For this review, take the finished solid that the model builds, in its own axes (mm). Face numbers are marked on the shaded views. Round coordinates to 2 decimals unless told otherwise and drop trailing zeros. Loops run counter-clockwise (first coordinate to the right, second up) from the corner with the lowest first, then second, coordinate; pieces in that order, holes last.
```python
from build123d import *

# Parameters (mm, degrees)
F0_R      = 0.381
F1_DEPTH  = 6.096
F2_SIZE2  = 0.3666174209
F2_SIZE   = 0.635
F0_R_2    = 1.1811
F1_FACE_R = 0.381
F3_DEPTH  = 0.762
F4_R      = 0.762
F4_R_2    = 0.508
F5_DEPTH  = 2.413
F6_R      = 1.1811
F6_R_2    = 0.762
F6_R_3    = 0.508
F7_DEPTH  = 0.762


with BuildPart() as f1:
    # F0 (on Top) → F1 (new body)
    with BuildSketch(Plane.XY):
        Circle(F0_R)
    extrude(amount=-F1_DEPTH)

    # F2
    f2_edges = [f1.edges().sort_by_distance(p)[0] for p in [
        (-0.381, 0, -6.096),
    ]]
    f2_side = f1.faces().sort_by_distance((-0.381, 0, -3.048))[0]
    chamfer(f2_edges, length=F2_SIZE, length2=F2_SIZE2, reference=f2_side)

    # F0 (on Top) + F1_face (on face) → F3 (join)
    with BuildSketch(Plane.XY):
        Circle(F0_R_2)
        Circle(F0_R, mode=Mode.SUBTRACT)
    with BuildSketch(Plane.XY):
        Circle(F1_FACE_R)
    extrude(amount=F3_DEPTH)

    # F4 (on face) → F5 (join)
    with BuildSketch(Plane.XY.offset(0.762)):
        Circle(F4_R)
        Circle(F4_R_2, mode=Mode.SUBTRACT)
    extrude(amount=F5_DEPTH)

    # F6 (on face) → F7 (join)
    with BuildSketch(Plane.XY.offset(3.175)):
        Circle(F6_R)
        Circle(F6_R_2, mode=Mode.SUBTRACT)
        Circle(F6_R_2)
        Circle(F6_R_3, mode=Mode.SUBTRACT)
    extrude(amount=F7_DEPTH)


solid = f1.part
```
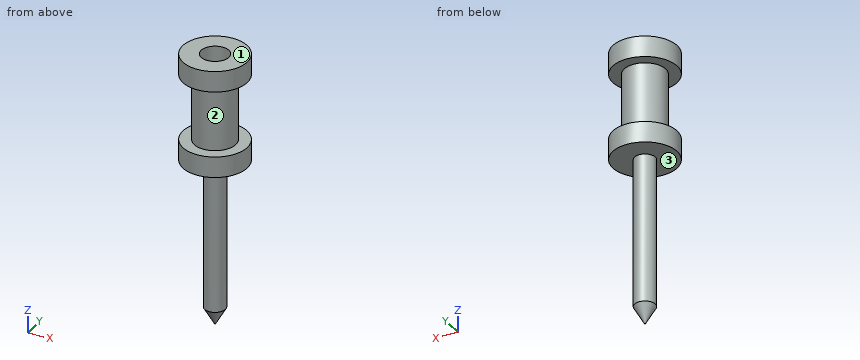
(1) Add section C-C (x = -0.9). Give the boundary of the cut face in (y, z) (3 decimals).
(2) Add section B-B (z = 3.5). Give the boundary of the cut face in (x, y).
(3) Add section D-D (z = -2.5). Give the boundary of the cut face in (x, y).
(4) The part is to be moulded in two halves that separate along Z. For the marked faces 1, 2 and 3, say which applies: pulls with the +Z half, pulls with the -Z half, needs draft (parallel to the pull), parting line crosses it, or undercut.
(5) Insertion check: pin 1 Ø0.7 at (x, y) = (0.5, 0) entering from -Z. The pin has a flat end and moves straight along its axis. Give the tip position at first contact, or say it passes through.
(6) Add section A-A (y = 0.85). Give the boundary of the cut face in (x, z) (3 decimals).
(7) For L1, parallel to Z at x = -0.95, y = -0.3 (3 decimals); L2, parallel to Y at x = 0, z = 2.1; L3, parallel to Z at x = 0, y = -0.65, list the stretches that pass through material, from the lowest coordinate up.
Outcome:
1. outline: (-0.765, 0) - (0.765, 0) - (0.765, 0.762) - (-0.765, 0.762) - close; (-0.765, 3.175) - (0.765, 3.175) - (0.765, 3.937) - (-0.765, 3.937) - close
2. outline: circle Ø2.36 at (0, 0); hole circle Ø1.02 at (0, 0)
3. outline: circle Ø0.76 at (0, 0)
4. face 1: pulls with the +Z half
4. face 2: undercut
4. face 3: pulls with the -Z half
5. pin 1: stops at z = -5.86
6. outline: (-0.82, 0) - (0.82, 0) - (0.82, 0.762) - (-0.82, 0.762) - close; (-0.82, 3.175) - (0.82, 3.175) - (0.82, 3.937) - (-0.82, 3.937) - close
7. L1: z = 0 to 0.762, 3.175 to 3.937
7. L2: y = -0.76 to -0.51, 0.51 to 0.76
7. L3: z = 0 to 3.94
